```python
from build123d import *

# Parameters (mm, degrees)
PAD003_DEPTH    = 5
PAD_DEPTH       = 3.25
POCKET012_DEPTH = 54.7
FILLET_R        = 1.5
PAD004_DEPTH    = 19.4
PAD005_DEPTH    = 2.1
PAD001_DEPTH    = 53.3
PAD002_DEPTH    = 53.3
POCKET_DEPTH    = 17.8
POCKET001_DEPTH = 5
POCKET011_DEPTH = 4
FILLET001_R     = 2


with BuildPart() as body:
    # Sketch025 → Pad003 (new body, symmetric)
    with BuildSketch(Plane.XZ):
        with BuildLine():
            Line((-64.25, 2.1), (-62.062493, 4.706969))
            ThreePointArc((-60.147382, 5.6), (-61.203928, 5.365769), (-62.062493, 4.706969))
            Line((-60.147382, 5.6), (-53.45, 5.6))
            Line((-53.45, 5.6), (-53.45, 4.6))
            Line((-53.45, 4.6), (-53.7, 4.6))
            Line((-54.7, 4.6), (-53.7, 4.6))
            Line((-54.7, 4.6), (-60.263959, 4.6))
            ThreePointArc((-60.263959, 4.6), (-60.792232, 4.482885), (-61.221515, 4.153485))
            Line((-61.221515, 4.153485), (-62.944593, 2.1))
            Line((-64.25, 2.1), (-62.944593, 2.1))
        make_face()
    extrude(amount=PAD003_DEPTH, both=True)

    # Sketch028 → Pad (join, symmetric)
    with BuildSketch(Plane.XZ):
        with BuildLine():
            Line((-53.7, 3.1), (-53.7, -6.209252))
            ThreePointArc((-53.7, -6.209252), (-53.653109, -6.384252), (-53.525, -6.512361))
            Line((-53.2, -6.7), (-53.525, -6.512361))
            Line((-53.2, -7.7), (-53.2, -6.7))
            ThreePointArc((-54.7, -6.103128), (-54.26619, -7.198573), (-53.2, -7.7))
            Line((-54.7, 3.1), (-54.7, -6.103128))
            Line((-54.7, 3.1), (-54.7, 4.6))
            Line((-54.7, 4.6), (-53.7, 4.6))
            Line((-53.7, 3.1), (-53.7, 4.6))
        make_face()
    extrude(amount=PAD_DEPTH, both=True)

    # Sketch027 → Pocket012 (cut)
    with BuildSketch(Plane.YZ):
        Polygon((3.25, -3.7), (0.940599, -7.7), (3.25, -7.7), align=None)
    pocket012 = extrude(amount=-POCKET012_DEPTH, mode=Mode.SUBTRACT)

    # Mirrored001: Pocket012 across Sketch027 V_Axis
    add(pocket012.mirror(Plane(origin=(0, 0, 0), x_dir=(1, 0, 0), z_dir=(0, 1, 0))), mode=Mode.SUBTRACT)

    # Fillet
    fillet_edges = [body.edges().sort_by_distance(p)[0] for p in [
        (-53.45, -5, 5.1),
        (-53.45, 5, 5.1),
    ]]
    fillet(fillet_edges, radius=FILLET_R)


with BuildPart() as body002:
    # Sketch011 → Pad004 (new body)
    with BuildSketch(Plane.XY):
        with BuildLine():
            Line((50.3, 5.5), (50.3, -5.5))
            ThreePointArc((50.3, -5.5), (50.885786, -6.914214), (52.3, -7.5))
            Line((53.3, -7.5), (52.3, -7.5))
            Line((53.3, -7.5), (55.6, -9.8))
            Line((55.6, 9.8), (55.6, -9.8))
            Line((53.3, 7.5), (55.6, 9.8))
            Line((52.3, 7.5), (53.3, 7.5))
            ThreePointArc((52.3, 7.5), (50.885786, 6.914214), (50.3, 5.5))
        make_face()
    extrude(amount=-PAD004_DEPTH)

    # Sketch029 → Pad005 (join)
    with BuildSketch(Plane.XY):
        with BuildLine():
            Line((50.3, 5.5), (50.3, -5.5))
            ThreePointArc((50.3, -5.5), (50.885786, -6.914214), (52.3, -7.5))
            Line((53.3, -7.5), (52.3, -7.5))
            Line((53.3, -7.5), (54.3, -7.5))
            ThreePointArc((54.3, -7.5), (55.714214, -6.914214), (56.3, -5.5))
            Line((56.3, 5.5), (56.3, -5.5))
            ThreePointArc((56.3, 5.5), (55.714214, 6.914214), (54.3, 7.5))
            Line((53.3, 7.5), (54.3, 7.5))
            Line((52.3, 7.5), (53.3, 7.5))
            ThreePointArc((52.3, 7.5), (50.885786, 6.914214), (50.3, 5.5))
        make_face()
    extrude(amount=PAD005_DEPTH)


with BuildPart() as obj1:
    # Sketch001 → Pad001 (new body, symmetric)
    with BuildSketch(Plane.XZ):
        Polygon((64.25, 0), (55.6, 0), (55.6, -19.4), (-55.6, -19.4), (-55.6, 0), (-64.25, 0), (-64.25, 2.1), (-53.3, 2.1), (-53.3, -16.9), (0, -16.9), (53.3, -16.9), (53.3, 2.1), (64.25, 2.1), align=None)
    extrude(amount=PAD001_DEPTH, both=True)

    # Sketch002 → Pad002 (join, symmetric)
    with BuildSketch(Plane.XZ):
        with BuildLine():
            ThreePointArc((52.9, 2.1), (52.15, 1.35), (52.9, 0.6))
            Line((53.3, 0.6), (52.9, 0.6))
            Line((53.3, 2.1), (53.3, 0.6))
            Line((53.3, 2.1), (52.9, 2.1))
        make_face()
    pad002 = extrude(amount=PAD002_DEPTH, both=True)

    # Sketch003 → Pocket (cut)
    with BuildSketch(Plane.XY):
        with BuildLine():
            ThreePointArc((28.8, 39.3), (40.3, 27.8), (51.8, 39.3))
            Line((51.8, 39.3), (51.8, 48.3))
            ThreePointArc((51.8, 48.3), (51.214214, 49.714214), (49.8, 50.3))
            Line((30.8, 50.3), (49.8, 50.3))
            ThreePointArc((30.8, 50.3), (29.385786, 49.714214), (28.8, 48.3))
            Line((28.8, 39.3), (28.8, 48.3))
        make_face()
        with BuildLine():
            ThreePointArc((51.8, -39.3), (40.3, -27.8), (28.8, -39.3))
            Line((28.8, -39.3), (28.8, -48.3))
            ThreePointArc((28.8, -48.3), (29.385786, -49.714214), (30.8, -50.3))
            Line((30.8, -50.3), (49.8, -50.3))
            ThreePointArc((49.8, -50.3), (51.214214, -49.714214), (51.8, -48.3))
            Line((51.8, -39.3), (51.8, -48.3))
        make_face()
    pocket = extrude(amount=-POCKET_DEPTH, mode=Mode.SUBTRACT)

    # Sketch004 → Pocket001 (cut)
    with BuildSketch(Plane.XY):
        with BuildLine():
            ThreePointArc((59.35, -45.8), (59.603187, -46.603007), (60.271172, -47.11557))
            Line((60.271172, -47.11557), (64.25, -48.563745))
            Line((64.25, -42.886255), (64.25, -48.563745))
            Line((60.271172, -44.33443), (64.25, -42.886255))
            ThreePointArc((60.271172, -44.33443), (59.603187, -44.846993), (59.35, -45.65))
            Line((59.35, -45.65), (59.35, -45.8))
        make_face()
        with BuildLine():
            ThreePointArc((60.471172, 47.11557), (59.803187, 46.603007), (59.55, 45.8))
            Line((59.55, 45.8), (59.55, 45.65))
            ThreePointArc((59.55, 45.65), (59.803187, 44.846993), (60.471172, 44.33443))
            Line((60.471172, 44.33443), (64.25, 42.959049))
            Line((64.25, 48.490951), (64.25, 42.959049))
            Line((60.471172, 47.11557), (64.25, 48.490951))
        make_face()
    pocket001 = extrude(amount=POCKET001_DEPTH, mode=Mode.SUBTRACT)

    # Mirrored: Pad002, Pocket, Pocket001 across Sketch002 V_Axis
    add(pad002.mirror(Plane(origin=(0, 0, 0), x_dir=(0, -1, 0), z_dir=(1, 0, 0))))
    add(pocket.mirror(Plane(origin=(0, 0, 0), x_dir=(0, -1, 0), z_dir=(1, 0, 0))), mode=Mode.SUBTRACT)
    add(pocket001.mirror(Plane(origin=(0, 0, 0), x_dir=(0, -1, 0), z_dir=(1, 0, 0))), mode=Mode.SUBTRACT)

    # Sketch024 → Pocket011 (cut, symmetric)
    with BuildSketch(Plane.XZ):
        with BuildLine():
            Line((-54.9, 3), (-54.9, -6.248633))
            ThreePointArc((-54.9, -6.248633), (-54.463, -7.367173), (-53.383476, -7.893225))
            Line((-53.383476, -7.893225), (-53.3, -7.9))
            Line((-51.9, 3), (-53.3, -7.9))
            Line((-54.9, 3), (-51.9, 3))
        make_face()
    extrude(amount=POCKET011_DEPTH, both=True, mode=Mode.SUBTRACT)

    # Boolean: union Body
    add(body.part)

    # Boolean001: cut Body002
    add(body002.part, mode=Mode.SUBTRACT)

    # Fillet001
    fillet001_edges = [obj1.edges().sort_by_distance(p)[0] for p in [
        (64.25, -53.3, 1.05),
        (64.25, 53.3, 1.05),
        (-64.25, -53.3, 1.05),
        (-64.25, 53.3, 1.05),
    ]]
    fillet(fillet001_edges, radius=FILLET001_R)


solid = obj1.part
```
Source: CAD feature listing. Evaluate the final solid. Frame: model axes, mm. A direction names the side the tool comes from. Round coordinates to 2 decimals unless told otherwise and drop trailing zeros. Loops run counter-clockwise (first coordinate to the right, second up) from the corner with the lowest first, then second, coordinate; pieces in that order, holes last. Notation, with made-up numbers: M 12.25,23.5 L 33.25,23.5 A10 ccw 33.25,38.5 Z; hole C 84.5,80.25 d6. An arc over 180 degrees is marked long. Put each result on its own line as item: value.
(1) Section A-A, the plane z = -1.5. Return loops of the section in (x, y), and give its area (3 significant figures).
Solutions:
outline: M -55.6,-53.3 L -53.3,-53.3 L -53.3,-4 L -54.9,-4 L -54.9,4 L -53.3,4 L -53.3,53.3 L -55.6,53.3 Z; M -54.7,-3.25 L -53.7,-3.25 L -53.7,3.25 L -54.7,3.25 Z; M 53.3,-53.3 L 55.6,-53.3 L 55.6,-9.8 L 53.3,-7.5 Z; M 53.3,7.5 L 55.6,9.8 L 55.6,53.3 L 53.3,53.3 Z
area: 444 mm²
(2) Pull-direction query (X, two-part tool) for faces 4 (the face through (40.047, 27.803, -17.344)), 5 (the face through (60, -1, 0)), 6 (the face through (55.6, -32, -10)), 7 (the face through (53.3, 30, -8)); classes: released by +X, released by -X, zero draft, split by the parting line, or undercut.
Solutions:
face 4: undercut
face 5: zero draft
face 6: released by +X
face 7: undercut
(3) Access query for faces 1 (the face through (-54.7, 0, -1)), 2 (the face through (-40, -39, -17.8)), 3 (the face through (-60, -1, 0)). Directions: +Z, -Z, +X, -X, +Y, -Y. A direction counts if a zero-diameter tool reaches every point of the face in a straight line with its end or side. Return the directions, or none.
Solutions:
face 1: none
face 2: +Z
face 3: -Z, -X, +Y, -Y
(4) First-contact query: pin 1 (2 mm diameter, centred on y = 41, z = -8, fed in from +X); pin 2 (9 mm diameter, centred on y = 31, z = -12.5, fed in from -X); pin 3 (7 mm diameter, centred on x = 37.5, y = -36.5, fed in from +Z). Flat tips, straight axial feed; report the tip coordinate or a pass-through.
Solutions:
pin 1: x = 55.6
pin 2: x = -55.6
pin 3: z = -17.8
(5) Section D-D, the plane x = 40.3. Return loops of the section in (y, z), and give its area (3 significant figures).
Solutions:
outline: M -53.3,-19.4 L 53.3,-19.4 L 53.3,-16.9 L 50.3,-16.9 L 50.3,-17.8 L 27.8,-17.8 L 27.8,-16.9 L -27.8,-16.9 L -27.8,-17.8 L -50.3,-17.8 L -50.3,-16.9 L -53.3,-16.9 Z
area: 226 mm²
(6) Section B-B, the plane y = -24. Return loops of the section in (x, z), and give its area (3 significant figures).
Solutions:
outline: M -64.25,0 L -55.6,0 L -55.6,-19.4 L 55.6,-19.4 L 55.6,0 L 64.25,0 L 64.25,2.1 L 52.9,2.1 A0.75 ccw 52.9,0.6 L 53.3,0.6 L 53.3,-16.9 L -53.3,-16.9 L -53.3,0.6 L -52.9,0.6 A0.75 ccw -52.9,2.1 L -64.25,2.1 Z
area: 405 mm²
(7) Section C-C, the plane z = -11.75. Return loops of the section in (x, y).
Solutions:
outline: M -55.6,-53.3 L -53.3,-53.3 L -53.3,53.3 L -55.6,53.3 Z; M 53.3,-53.3 L 55.6,-53.3 L 55.6,-9.8 L 53.3,-7.5 Z; M 53.3,7.5 L 55.6,9.8 L 55.6,53.3 L 53.3,53.3 Z
(8) Ray query, line 1 (X direction, y = 17, z = -2.5); line 2 (Z direction, x = -14, y = 28.5); line 3 (Z direction, x = 53.5, y = -22). Return the intervals inside material, ascending. Write a range as [from, to].
Solutions:
line 1: [-55.6, -53.3], [53.3, 55.6]
line 2: [-19.4, -16.9]
line 3: [-19.4, 2.1]
